Here's the drawing with two shaded views (mm, measured from the low corner). I have some questions. A direction names the side the tool comes from. Coordinates: 2 decimals unless noted, no trailing zeros. Write each loop counter-clockwise with the first axis right and the second up, starting at its lowest first coordinate (ties: lowest second). Pieces come first, ordered by that corner, then holes. Notation, with made-up numbers: (-12, 12.25) -> (8, 12.25) arc R25 ccw to (8, 29.25) -> close; hole circle Ø4 at (21.25, -1). An arc over 180 degrees is marked (long way). Use one line per item in the form item = value.
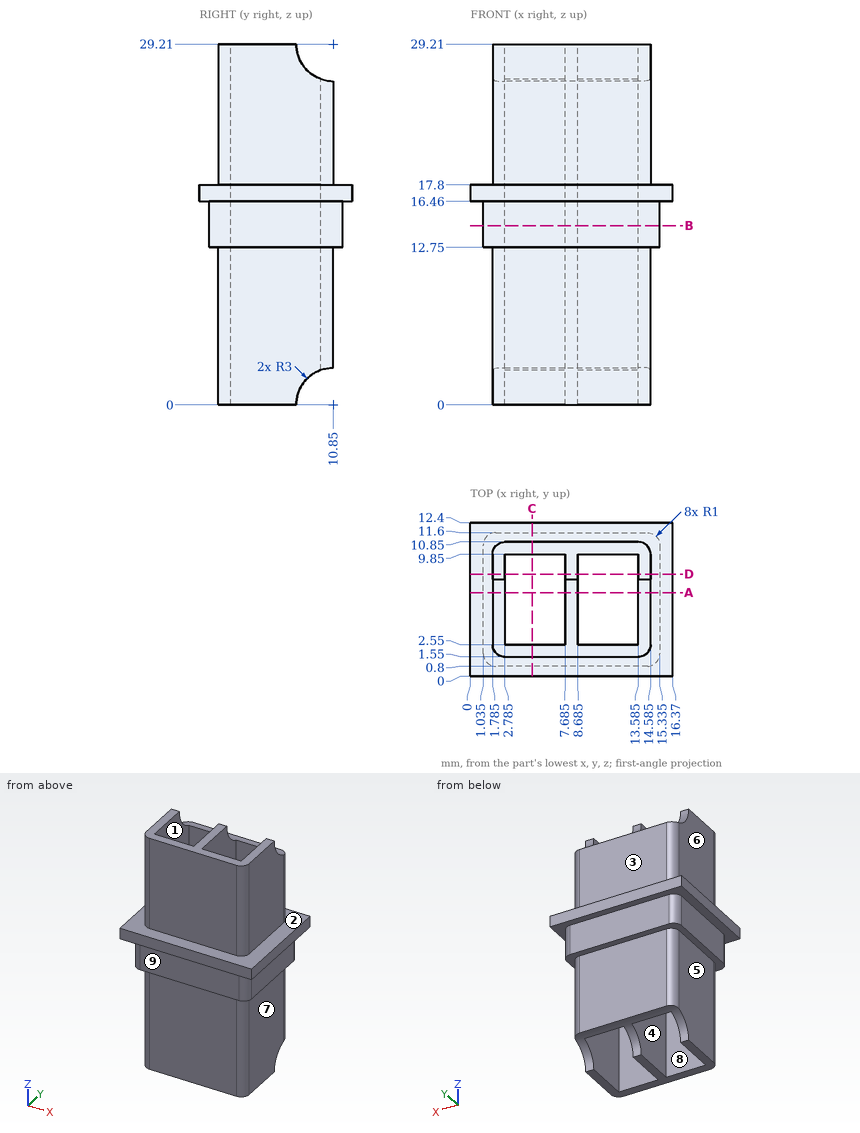
Q1. Suppose I cut it at A-A (y = 6.75). Write out the boundary of the cut face in (x, z) (3 decimals).
Return value:
outline = (0, 16.46) -> (1.035, 16.46) -> (1.035, 12.75) -> (1.785, 12.75) -> (1.785, 0) -> (2.785, 0) -> (2.785, 29.21) -> (1.785, 29.21) -> (1.785, 17.8) -> (0, 17.8) -> close; (7.685, 0) -> (8.685, 0) -> (8.685, 29.21) -> (7.685, 29.21) -> close; (13.585, 0) -> (14.585, 0) -> (14.585, 12.75) -> (15.335, 12.75) -> (15.335, 16.46) -> (16.37, 16.46) -> (16.37, 17.8) -> (14.585, 17.8) -> (14.585, 29.21) -> (13.585, 29.21) -> close
Q2. Suppose I cut it at D-D (y = 8.25). Write out the boundary of the cut face in (x, z) (3 decimals), then the cut area to 3 significant figures.
Return value:
outline = (0, 16.46) -> (1.035, 16.46) -> (1.035, 12.75) -> (1.785, 12.75) -> (1.785, 1.497) -> (2.785, 1.497) -> (2.785, 27.713) -> (1.785, 27.713) -> (1.785, 17.8) -> (0, 17.8) -> close; (7.685, 1.497) -> (8.685, 1.497) -> (8.685, 27.713) -> (7.685, 27.713) -> close; (13.585, 1.497) -> (14.585, 1.497) -> (14.585, 12.75) -> (15.335, 12.75) -> (15.335, 16.46) -> (16.37, 16.46) -> (16.37, 17.8) -> (14.585, 17.8) -> (14.585, 27.713) -> (13.585, 27.713) -> close
area = 89.0 mm2
Q3. Will these pins go through, and if not, where does the flat tip stop? pin 1 (3 mm diameter, centred on x = 13.5, z = 8.5, fed in from +Y); pin 2 (6 mm diameter, centred on y = 4.5, z = 23.5, fed in from -X) (3 decimals); pin 3 (2.5 mm diameter, centred on x = 5, z = 15, fed in from +Y).
Return value:
pin_1 = 10.85
pin_2 = 1.785
pin_3 = 11.6
Q4. If I drill on line 1 (X direction, y = 6.25, z = 7.25) (3 decimals); line 2 (X direction, y = 8, z = 16.5) (3 decimals); line 3 (Y direction, x = 3.75, z = 6.25), over which ranges is the centre line in solid material (lowest first)? Write a range as from..to.
Return value:
line_1 = 1.785..2.785, 7.685..8.685, 13.585..14.585
line_2 = 0..2.785, 7.685..8.685, 13.585..16.37
line_3 = 1.55..2.55, 9.85..10.85
Q5. Suppose I cut it at B-B (z = 14.5). Write out the boundary of the cut face in (x, y) (3 decimals).
Return value:
outline = (1.035, 1.8) arc R1 ccw to (2.035, 0.8) -> (14.335, 0.8) arc R1 ccw to (15.335, 1.8) -> (15.335, 10.6) arc R1 ccw to (14.335, 11.6) -> (2.035, 11.6) arc R1 ccw to (1.035, 10.6) -> close; hole (2.785, 2.55) -> (7.685, 2.55) -> (7.685, 9.85) -> (2.785, 9.85) -> close; hole (8.685, 2.55) -> (13.585, 2.55) -> (13.585, 9.85) -> (8.685, 9.85) -> close
Q6. For the marked faces 5, 6, 7, 8 and 9, which set-ups out of +Z, -Z, +X, -X, +Y, -Y let a thin tool reach every point of the face, with its end or its side?
Return value:
face_5 = -Z, -X, +Y, -Y
face_6 = +Z, -X, +Y, -Y
face_7 = -Z, +X, +Y, -Y
face_8 = +Z, -Z
face_9 = -Z, +X, -X, -Y
Q7. Thinking about a two-plate mould opening in Y: for the marked faces 1, 2, 3 and 4, which applies, released by +Y, released by -Y, zero draft, split by the parting line, or undercut?
Return value:
face_1 = undercut
face_2 = zero draft
face_3 = released by +Y
face_4 = undercut
Q8. Suppose I cut it at C-C (x = 5). Write out the boundary of the cut face in (y, z), then the cut area to 3 significant figures.
Return value:
outline = (0, 16.46) -> (0.8, 16.46) -> (0.8, 12.75) -> (1.55, 12.75) -> (1.55, 0) -> (2.55, 0) -> (2.55, 29.21) -> (1.55, 29.21) -> (1.55, 17.8) -> (0, 17.8) -> close; (9.85, 2.83) arc R3 cw to (10.85, 3) -> (10.85, 12.75) -> (11.6, 12.75) -> (11.6, 16.46) -> (12.4, 16.46) -> (12.4, 17.8) -> (10.85, 17.8) -> (10.85, 26.21) arc R3 cw to (9.85, 26.38) -> close
area = 62.3 mm2
